Geometry check sheet. Reference: the model listing, model coordinates, mm. Face numbers are marked on the shaded views. Round coordinates to 2 decimals unless told otherwise and drop trailing zeros. Write each loop counter-clockwise with the first axis right and the second up, starting at its lowest first coordinate (ties: lowest second). Pieces come first, ordered by that corner, then holes. Notation, with made-up numbers: M 7.5,52.25 L 53.5,52.25 A30 cw 53.5,90.25 Z; hole C 33,77 d3. An arc over 180 degrees is marked long. Use a Markdown table: item, result.
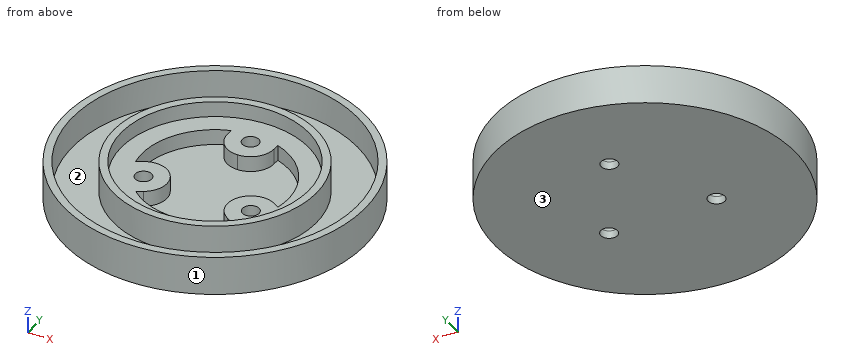
```python
from build123d import *

# Parameters (mm, degrees)
F0_R      = 38.5
F1_DEPTH  = 2
F2_R      = 38.5
F2_R_2    = 36.5
F3_DEPTH  = 8
F4_R      = 26
F4_R_2    = 24
F5_DEPTH  = 8
F6_R      = 24
F6_R_2    = 18.75
F7_DEPTH  = 4
F8_R      = 2.125
F9_DEPTH  = 12.5
F10_R     = 2.125
F11_DEPTH = 4
F12_R     = 5.99999


# Not quite as in the source:
# - a fillet or chamfer is up to 0.001 mm smaller than in the source, because OpenCascade refuses the exact size


with BuildPart() as f1:
    # F0 (on Top) → F1 (new body)
    with BuildSketch(Plane.XY):
        Circle(F0_R)
    extrude(amount=F1_DEPTH)

    # F2 (on face) → F3 (join)
    with BuildSketch(Plane.XY.offset(2)):
        Circle(F2_R)
        Circle(F2_R_2, mode=Mode.SUBTRACT)
    extrude(amount=F3_DEPTH)

    # F4 (on face) → F5 (join)
    with BuildSketch(Plane.XY.offset(2)):
        Circle(F4_R)
        Circle(F4_R_2, mode=Mode.SUBTRACT)
    extrude(amount=F5_DEPTH)

    # F6 (on face) → F7 (join)
    with BuildSketch(Plane.XY.offset(2)):
        Circle(F6_R)
        Circle(F6_R_2, mode=Mode.SUBTRACT)
    extrude(amount=F7_DEPTH)

    # F8 (on face) → F9 (cut, symmetric)
    with BuildSketch(Plane.XY.offset(2)):
        with Locations((0, 16)):
            Circle(F8_R)
        with Locations((-13.8564064606, -8)):
            Circle(F8_R)
        with Locations((13.8564064606, -8)):
            Circle(F8_R)
    extrude(amount=F9_DEPTH, both=True, mode=Mode.SUBTRACT)

    # F10 (on face) → F11 (join)
    with BuildSketch(Plane.XY.offset(2)):
        with BuildLine():
            Line((6, 16), (6, 17.7640789235))
            ThreePointArc((6, 17.7640789235), (0, 18.75), (-6, 17.7640789235))
            Line((-6, 17.7640789235), (-6, 16))
            Line((-6, 16), (-6, 10))
            Line((-6, 10), (0, 10))
            Line((0, 10), (6, 10))
            Line((6, 10), (6, 16))
        make_face()
        with Locations((0, 16)):
            Circle(F10_R, mode=Mode.SUBTRACT)
        with BuildLine():
            Line((-16.8564064606, -2.8038475773), (-18.3841436226, -3.685887039))
            ThreePointArc((-18.3841436226, -3.685887039), (-16.237976321, -9.375), (-12.3841436226, -14.0781918845))
            Line((-12.3841436226, -14.0781918845), (-10.8564064606, -13.1961524227))
            Line((-10.8564064606, -13.1961524227), (-5.6602540378, -10.1961524227))
            Line((-5.6602540378, -10.1961524227), (-8.6602540378, -5))
            Line((-8.6602540378, -5), (-11.6602540378, 0.1961524227))
            Line((-11.6602540378, 0.1961524227), (-16.8564064606, -2.8038475773))
        make_face()
        with Locations((-13.8564064606, -8)):
            Circle(F10_R, mode=Mode.SUBTRACT)
        with BuildLine():
            ThreePointArc((12.3841436226, -14.0781918845), (16.237976321, -9.375), (18.3841436226, -3.685887039))
            Line((18.3841436226, -3.685887039), (16.8564064606, -2.8038475773))
            Line((16.8564064606, -2.8038475773), (11.6602540378, 0.1961524227))
            Line((11.6602540378, 0.1961524227), (8.6602540378, -5))
            Line((8.6602540378, -5), (5.6602540378, -10.1961524227))
            Line((5.6602540378, -10.1961524227), (10.8564064606, -13.1961524227))
            Line((10.8564064606, -13.1961524227), (12.3841436226, -14.0781918845))
        make_face()
        with Locations((13.8564064606, -8)):
            Circle(F10_R, mode=Mode.SUBTRACT)
    extrude(amount=F11_DEPTH)

    # F12 (radius 6 in the source; OpenCascade refuses exactly that, so slightly less here)
    f12_edges = [f1.edges().sort_by_distance(p)[0] for p in [
        (-6, 10, 4),
        (6, 10, 4),
        (11.660254, 0.196152, 4),
        (5.660254, -10.196152, 4),
        (-5.660254, -10.196152, 4),
        (-11.660254, 0.196152, 4),
    ]]
    fillet(f12_edges, radius=F12_R)


solid = f1.part
```
Item 1: Cross-section at C-C, the plane y = -8. Record the cut outline in (x, z).
Outcome:
| item | result |
|---|---|
| outline | M -37.66,0 L -15.98,0 L -15.98,6 L -22.63,6 L -22.63,10 L -24.74,10 L -24.74,2 L -35.61,2 L -35.61,10 L -37.66,10 Z; M -11.73,0 L 11.73,0 L 11.73,6 L 7.86,6 L 7.86,2 L -7.86,2 L -7.86,6 L -11.73,6 Z; M 15.98,0 L 37.66,0 L 37.66,10 L 35.61,10 L 35.61,2 L 24.74,2 L 24.74,10 L 22.63,10 L 22.63,6 L 15.98,6 Z |
Item 2: Cross-section at B-B, the plane z = 7.75. Record the cut outline in (x, y).
Outcome:
| item | result |
|---|---|
| outline | C 0,0 d77; C 0,0 d52; hole C 0,0 d73; hole C 0,0 d48 |
Item 3: Cross-section at D-D, the plane x = -23. Record the cut outline in (y, z), and give its area (3 significant figures).
Outcome:
| item | result |
|---|---|
| outline | M -30.87,0 L 30.87,0 L 30.87,10 L 28.34,10 L 28.34,2 L 12.12,2 L 12.12,10 L 6.86,10 L 6.86,6 L -6.86,6 L -6.86,10 L -12.12,10 L -12.12,2 L -28.34,2 L -28.34,10 L -30.87,10 Z |
| area | 303 mm2 |
Item 4: Cross-section at A-A, the plane z = 3.5. Count the separate pieces of the cut face and the enclosed holes in it, and give its area (3 significant figures).
Outcome:
| item | result |
|---|---|
| separate pieces | 2 |
| enclosed holes | 5 |
| area | 1,700 mm2 |
Item 5: Material ranges on line 1 along Y through (x, z) = (0, 3.9) (3 decimals); line 2 along Y through (x, z) = (0, 1.45) (3 decimals); line 3 along Y through (x, z) = (23.5, 4), recorded low to high. Write a range as from..to.
Outcome:
| item | result |
|---|---|
| line 1 | y = -38.5..-36.5, -26..-18.75, 10..13.875, 18.125..26, 36.5..38.5 |
| line 2 | y = -38.5..13.875, 18.125..38.5 |
| line 3 | y = -30.5..-27.93, -11.12..11.12, 27.93..30.5 |
Item 6: Go/stop test with flat-tipped pins: pin 1 (3 mm diameter, centred on y = -28.5, z = 6.5, fed in from +X); pin 2 (7 mm diameter, centred on x = 0, y = 16, fed in from +Z); pin 3 (1.9 mm diameter, centred on y = 16.5, z = 5, fed in from +X). Record where each tip stops, or that it passes through.
Outcome:
| item | result |
|---|---|
| pin 1 | stops at x = 27.45 |
| pin 2 | stops at z = 6 |
| pin 3 | stops at x = 35.22 |
Item 7: Mould release check, pull along X, two halves, no side actions. Record for the marked faces 1, 2 and 3: +X half, -X half, draft (parallel to the pull), parting line (faces both ways), or undercut.
Outcome:
| item | result |
|---|---|
| face 1 | parting line |
| face 2 | undercut |
| face 3 | draft |
